Check sheet for the modelled part. Datum: model origin and axes. Units: mm. A direction names the side the tool comes from. Round coordinates to 2 decimals unless told otherwise and drop trailing zeros. Loops run counter-clockwise (first coordinate to the right, second up) from the corner with the lowest first, then second, coordinate; pieces in that order, holes last. Notation, with made-up numbers: M 10,56.25 L 23,56.25 A13 cw 23,74.25 Z; hole C 17.25,-33 d8. An arc over 180 degrees is marked long. One line per question, with ' | ' between items. Start each with the question number.
(1) Draft check along Y on faces 1 (the face through (0.34, 11.12, 4.93)), 2 (the face through (-3, -9, 10)), 3 (the face through (-1.978, -8.908, 4.93)). Enter one of: +Y half, -Y half, draft (parallel to the pull), parting line (faces both ways), or undercut.
(2) Thickness scan on probe 1 along Y at (x, z) = (0, 4) (3 decimals); probe 2 along X at (y, z) = (0.5, 1); probe 3 along X at (y, z) = (5.5, 8.25). Record the ranges inside material, lowest first. Write a range as [from, to].
(3) Go/stop test with flat-tipped pins: P1, Ø1, axis at y = -4, z = 4, coming from the -X side; P2, Ø4, axis at y = -8.5, z = 6.5, coming from the +X side (3 decimals); P3, Ø2.5, axis at y = -8.5, z = 6, coming from the -X side (3 decimals); P4, Ø5, axis at x = 3.5, y = 3.5, coming from the -Z side. Record where each tip stops, or that it passes through.
(4) Tool access check on faces 4 (the face through (-9.125, -9, 5)), 5 (the face through (9.125, -9, 5)), 6 (the face through (0, -11.125, 5)). Record the directions out of +Z, -Z, +X, -X, +Y, -Y that give a thin tool (end or side, any length) a straight path to the whole face; none if there is none.
(5) Section check C-C (z = 5.5). Record the boundary of the cut face in (x, y) (3 decimals).
(6) Section check A-A (x = 0). Record the boundary of the cut face in (y, z) (3 decimals).
```python
from build123d import *

# Parameters (mm, degrees)
SKETCH1_R           = 11.125
SKETCH1_R_2         = 9.125
BOSS_EXTRUDE1_DEPTH = 10
BOSS_EXTRUDE2_START = -10
BOSS_EXTRUDE2_DEPTH = 10


with BuildPart() as part:
    # Sketch1 → Boss-Extrude1 (new body)
    with BuildSketch(Plane.XY):
        Circle(SKETCH1_R)
        Circle(SKETCH1_R_2, mode=Mode.SUBTRACT)
    extrude(amount=BOSS_EXTRUDE1_DEPTH)

    # Sketch2 → Boss-Extrude2 (add)
    with BuildSketch(Plane.XY.offset(10).offset(BOSS_EXTRUDE2_START)):
        with BuildLine():
            Line((-9.125, -9.125), (-6.363961031, -9.125))
            ThreePointArc((-6.363961031, -9.125), (-7.866562941, -7.866562941), (-9.125, -6.363961031))
            Line((-9.125, -6.363961031), (-9.125, -9.125))
        make_face()
        with BuildLine():
            Line((-9.125, -11.125), (0, -11.125))
            ThreePointArc((0, -11.125), (-3.335416016, -10.613228774), (-6.363961031, -9.125))
            Line((-6.363961031, -9.125), (-9.125, -9.125))
            Line((-9.125, -9.125), (-9.125, -11.125))
        make_face()
        with BuildLine():
            Line((0, -11.125), (9.125, -11.125))
            Line((9.125, -11.125), (9.125, -9.125))
            Line((9.125, -9.125), (6.363961031, -9.125))
            ThreePointArc((6.363961031, -9.125), (3.335416016, -10.613228774), (0, -11.125))
        make_face()
        with BuildLine():
            Line((6.363961031, -9.125), (9.125, -9.125))
            Line((9.125, -9.125), (9.125, -6.363961031))
            ThreePointArc((9.125, -6.363961031), (7.866562941, -7.866562941), (6.363961031, -9.125))
        make_face()
    extrude(amount=BOSS_EXTRUDE2_DEPTH)


solid = part.part
```
The answers:
1) face 1: parting line | face 2: draft | face 3: undercut
2) probe 1: [-11.125, -9.125], [9.125, 11.125] | probe 2: [-11.11, -9.11], [9.11, 11.11] | probe 3: [-9.67, -7.28], [7.28, 9.67]
3) P1: x = -10.56 | P2: x = 9.125 | P3: x = -9.125 | P4: through
4) face 4: +Z, -Z, -X, -Y | face 5: +Z, -Z, +X, -Y | face 6: +Z, -Z, +X, -X, -Y
5) outline: M -9.125,-11.125 L 9.125,-11.125 L 9.125,-6.364 A11.125 ccw long -9.125,-6.364 Z; hole C 0,0 d18.25
6) outline: M -11.125,0 L -9.125,0 L -9.125,10 L -11.125,10 Z; M 9.125,0 L 11.125,0 L 11.125,10 L 9.125,10 Z
